Drawing for the job (mm, zero at the part's lowest x, y, z). A direction names the side the tool comes from. Give positions to 0.01 mm unless a question says otherwise; leave off trailing zeros. Order: outer loops, then holes, each group sorted by start corner. A loop starts at its lowest first (then second) coordinate and runs counter-clockwise, first axis right, second up. Notation, with made-up numbers: (9.25, 18.5) - (22.25, 18.5) arc R13 ccw to (22.25, 43.5) - close; hole circle Ø7 at (-9, 37.5). An arc over 180 degrees is marked (long way). Use a Markdown table: item, result.
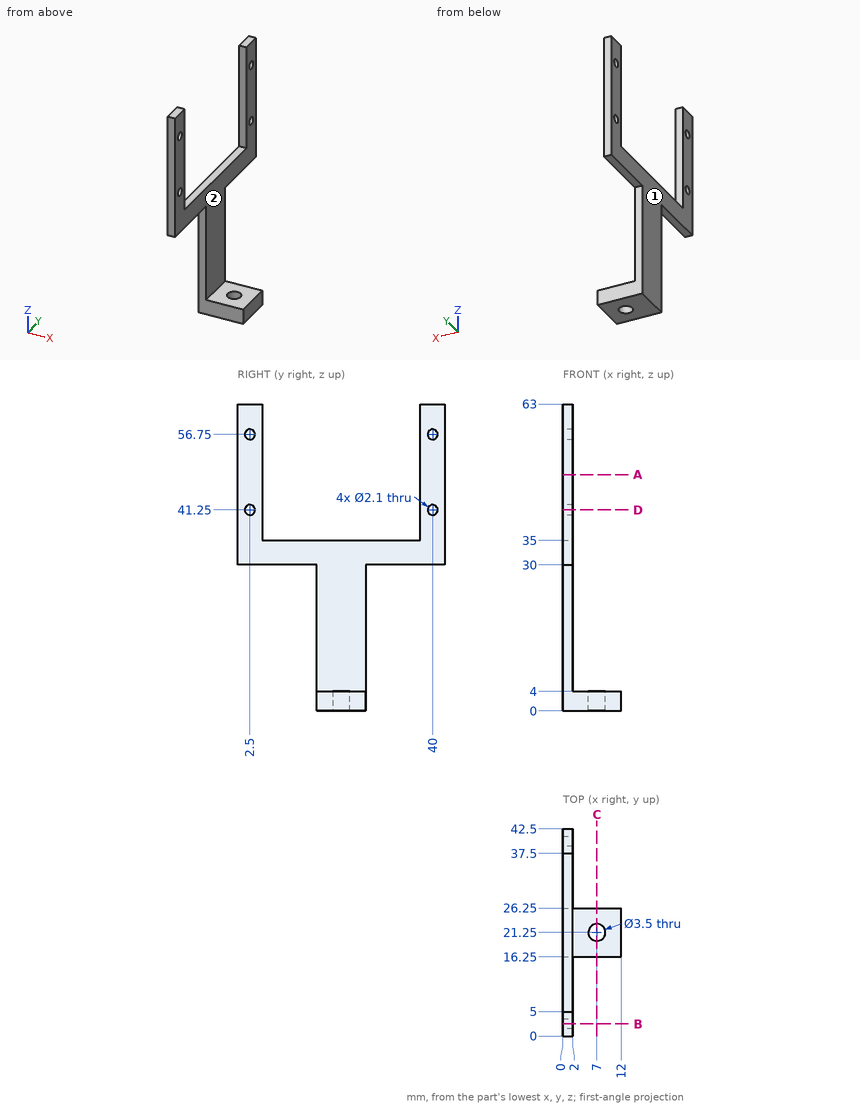
1) Slice it at B-B (y = 2.5). Write the cut outline in (x, z).
Computed:
| item | result |
|---|---|
| outline | (0, 30) - (2, 30) - (2, 40.2) - (0, 40.2) - close; (0, 42.3) - (2, 42.3) - (2, 55.7) - (0, 55.7) - close; (0, 57.8) - (2, 57.8) - (2, 63) - (0, 63) - close |
2) Slice it at A-A (z = 48.5). Write the cut outline in (x, y), and give its area (3 significant figures).
Computed:
| item | result |
|---|---|
| outline | (0, 0) - (2, 0) - (2, 5) - (0, 5) - close; (0, 37.5) - (2, 37.5) - (2, 42.5) - (0, 42.5) - close |
| area | 20.0 mm² |
3) Pin check, flat tips, straight feed: P1, Ø4.5, axis at x = 7, y = 21.25, coming from the -Z side; P2, Ø12, axis at y = 6.5, z = 44.5, coming from the +X side; P3, Ø1, axis at x = 1, y = 36.5, coming from the -Z side; P4, Ø1, axis at x = 1.5, y = 20, coming from the +Z side. Stop position of each tip, or through.
Computed:
| item | result |
|---|---|
| P1 | stops at z = 0 |
| P2 | stops at x = 2 |
| P3 | stops at z = 30 |
| P4 | stops at z = 35 |
4) Slice it at D-D (z = 41.25). Write the cut outline in (x, y).
Computed:
| item | result |
|---|---|
| outline | (0, 0) - (2, 0) - (2, 1.45) - (0, 1.45) - close; (0, 3.55) - (2, 3.55) - (2, 5) - (0, 5) - close; (0, 37.5) - (2, 37.5) - (2, 38.95) - (0, 38.95) - close; (0, 41.05) - (2, 41.05) - (2, 42.5) - (0, 42.5) - close |
5) Tool access for the marked faces 1 and 2: list every direction of +Z, -Z, +X, -X, +Y, -Y with a clear straight run to the whole face (end or side of a thin tool).
Computed:
| item | result |
|---|---|
| face 1 | +Z, -Z, -X, +Y, -Y |
| face 2 | +Z, +X, +Y, -Y |
6) Wall check: line 1 (Z direction, x = 1.4, y = 40); line 2 (Z direction, x = 1.5, y = 2); line 3 (X direction, y = 21.25, z = 0.8). Give the ranges that are in metal, low to high. Write a range as from..to.
Computed:
| item | result |
|---|---|
| line 1 | z = 30..40.2, 42.3..55.7, 57.8..63 |
| line 2 | z = 30..40.33, 42.17..55.83, 57.67..63 |
| line 3 | x = 0..5.25, 8.75..12 |
7) Slice it at C-C (x = 7). Write the cut outline in (y, z), and give its area (3 significant figures).
Computed:
| item | result |
|---|---|
| outline | (16.25, 0) - (19.5, 0) - (19.5, 4) - (16.25, 4) - close; (23, 0) - (26.25, 0) - (26.25, 4) - (23, 4) - close |
| area | 26.0 mm² |
